from build123d import *

# Parameters (mm, degrees)
BOSS_EXTRUDE1_DEPTH     = 1.3
SKETCH2_R               = 1.33
CUT_EXTRUDE1_DEPTH      = 36.818151823
MIRROR2_COPY_1_SKETCH_R = 1.33
MIRROR2_COPY_1_DEPTH    = 36.818151823
CUT_EXTRUDE2_DEPTH      = 0.1
SKETCH4_R               = 0.5
CUT_EXTRUDE3_DEPTH      = 36.814661802
LPATTERN1_COUNT         = 20
LPATTERN1_PITCH         = 2.54
LPATTERN1_COUNT_DIR2    = 2
LPATTERN1_PITCH_DIR2    = 2.5
SKETCH5_R               = 0.5
CUT_EXTRUDE4_DEPTH      = 36.814661802
LPATTERN2_COUNT         = 2
LPATTERN2_PITCH         = 2.54
LPATTERN2_COUNT_DIR2    = 2
LPATTERN2_PITCH_DIR2    = 2.5
SKETCH7_R               = 3
CUT_EXTRUDE5_DEPTH      = 0.1
MIRROR4_COPY_1_SKETCH_R = 3
MIRROR4_COPY_1_DEPTH    = 0.1
SKETCH8_W               = 12
SKETCH8_H               = 12
BOSS_EXTRUDE2_DEPTH     = 1.25
BOSS_EXTRUDE3_START     = -7.8
BOSS_EXTRUDE3_DEPTH     = 7.6
CUT_EXTRUDE6_DEPTH      = 7.25
BOSS_EXTRUDE4_START     = -10.5
BOSS_EXTRUDE4_DEPTH     = 5.75
CUT_EXTRUDE7_DEPTH      = 5.4
LPATTERN3_COUNT         = 2
LPATTERN3_PITCH         = 12.5
BOSS_EXTRUDE5_START     = 29.3
SKETCH14_W              = 1.2
SKETCH14_H              = 17
BOSS_EXTRUDE5_DEPTH     = 4.1


with BuildPart() as part:
    # Sketch1 → Boss-Extrude1 (new body)
    with BuildSketch(Plane.XY):
        with BuildLine():
            Line((-29, -15), (29, -15))
            ThreePointArc((29, -15), (31.474873734, -13.974873734), (32.5, -11.5))
            Line((32.5, -11.5), (32.5, 11.5))
            ThreePointArc((32.5, 11.5), (31.474873734, 13.974873734), (29, 15))
            Line((29, 15), (-29, 15))
            ThreePointArc((-29, 15), (-31.474873734, 13.974873734), (-32.5, 11.5))
            Line((-32.5, 11.5), (-32.5, -11.5))
            ThreePointArc((-32.5, -11.5), (-31.474873734, -13.974873734), (-29, -15))
        make_face()
    extrude(amount=BOSS_EXTRUDE1_DEPTH)

    # Sketch2 → Cut-Extrude1 (cut, through all)
    with BuildSketch(Plane.XY.offset(1.3)):
        with Locations((-28.75, 11.25)):
            Circle(SKETCH2_R)
    cut_extrude1 = extrude(amount=-CUT_EXTRUDE1_DEPTH, mode=Mode.SUBTRACT)

    # Mirror1: Cut-Extrude1 across plane
    add(cut_extrude1.mirror(Plane.ZX), mode=Mode.SUBTRACT)

    # Mirror2: Cut-Extrude1 across plane
    add(cut_extrude1.mirror(Plane(origin=(0, 0, 0), x_dir=(0, 0, 1), z_dir=(1, 0, 0))), mode=Mode.SUBTRACT)

    # Mirror2 copy 1 sketch → Mirror2 copy 1 (cut, through all)
    with BuildSketch(Plane(origin=(0, 0, 1.3), x_dir=(-1, 0, 0), z_dir=(0, 0, 1))):
        with Locations((-28.75, 11.25)):
            Circle(MIRROR2_COPY_1_SKETCH_R)
    extrude(amount=-MIRROR2_COPY_1_DEPTH, mode=Mode.SUBTRACT)

    # Sketch3 → Cut-Extrude2 (cut)
    with BuildSketch(Plane.XY.offset(1.3)):
        Polygon((-25.5, 14.3), (25.5, 14.3), (25.5, 4.2), (20.4, 4.2), (20.4, 9.2), (-25.5, 9.2), align=None)
    extrude(amount=-CUT_EXTRUDE2_DEPTH, mode=Mode.SUBTRACT)

    # Sketch4 → Cut-Extrude3 (cut, through all)
    with BuildSketch(Plane.XY.offset(1.2)):
        with Locations((-24.13, 13)):
            Circle(SKETCH4_R)
    cut_extrude3 = extrude(amount=-CUT_EXTRUDE3_DEPTH, mode=Mode.SUBTRACT)

    # LPattern1: Cut-Extrude3 20 × 2
    with Locations(*[(i * LPATTERN1_PITCH, -j * LPATTERN1_PITCH_DIR2, 0) for i in range(LPATTERN1_COUNT) for j in range(LPATTERN1_COUNT_DIR2) if (i, j) != (0, 0)]):
        add(cut_extrude3, mode=Mode.SUBTRACT)

    # Sketch5 → Cut-Extrude4 (cut, through all)
    with BuildSketch(Plane.XY.offset(1.2)):
        with Locations((21.59, 8)):
            Circle(SKETCH5_R)
    cut_extrude4 = extrude(amount=-CUT_EXTRUDE4_DEPTH, mode=Mode.SUBTRACT)

    # LPattern2: Cut-Extrude4 2 × 2
    with Locations(*[(i * LPATTERN2_PITCH, -j * LPATTERN2_PITCH_DIR2, 0) for i in range(LPATTERN2_COUNT) for j in range(LPATTERN2_COUNT_DIR2) if (i, j) != (0, 0)]):
        add(cut_extrude4, mode=Mode.SUBTRACT)

    # Sketch7 → Cut-Extrude5 (cut)
    with BuildSketch(Plane.XY.offset(1.3)):
        with Locations((-28.75, 11.25)):
            Circle(SKETCH7_R)
    cut_extrude5 = extrude(amount=-CUT_EXTRUDE5_DEPTH, mode=Mode.SUBTRACT)

    # Mirror3: Cut-Extrude5 across plane
    add(cut_extrude5.mirror(Plane.ZX), mode=Mode.SUBTRACT)

    # Mirror4: Cut-Extrude5 across plane
    add(cut_extrude5.mirror(Plane(origin=(0, 0, 0), x_dir=(0, 0, 1), z_dir=(1, 0, 0))), mode=Mode.SUBTRACT)

    # Mirror4 copy 1 sketch → Mirror4 copy 1 (cut)
    with BuildSketch(Plane(origin=(0, 0, 1.3), x_dir=(-1, 0, 0), z_dir=(0, 0, 1))):
        with Locations((-28.75, 11.25)):
            Circle(MIRROR4_COPY_1_SKETCH_R)
    extrude(amount=-MIRROR4_COPY_1_DEPTH, mode=Mode.SUBTRACT)

    # Sketch8 → Boss-Extrude2 (add)
    with BuildSketch(Plane.XY.offset(1.3)):
        with Locations((-6.7, -2)):
            Rectangle(SKETCH8_W, SKETCH8_H)
    extrude(amount=BOSS_EXTRUDE2_DEPTH)

    # Sketch9 → Boss-Extrude3 (add)
    with BuildSketch(Plane(origin=(0, 0, 0), x_dir=(1, 0, 0), z_dir=(0, 1, 0)).offset(BOSS_EXTRUDE3_START)):
        Polygon((-24.175, -1.3), (-15.575, -1.3), (-14.25, -2.76), (-14.25, -4.6), (-25.5, -4.6), (-25.5, -2.76), align=None)
    extrude(amount=-BOSS_EXTRUDE3_DEPTH)

    # Sketch10 → Cut-Extrude6 (cut)
    with BuildSketch(Plane.XZ.offset(15.4)):
        Polygon((-14.6, 2.895140858), (-14.6, 4.25), (-25.15, 4.25), (-25.15, 2.895140858), (-24.01999203, 1.65), (-15.73000797, 1.65), align=None)
    extrude(amount=-CUT_EXTRUDE6_DEPTH, mode=Mode.SUBTRACT)

    # Sketch12 → Boss-Extrude4 (add)
    with BuildSketch(Plane(origin=(0, 0, 0), x_dir=(1, 0, 0), z_dir=(0, 1, 0)).offset(BOSS_EXTRUDE4_START)):
        Polygon((17.8, -3.9), (25.35, -3.9), (25.35, -2.57), (24.125, -1.3), (19.025, -1.3), (17.8, -2.57), align=None)
    boss_extrude4 = extrude(amount=-BOSS_EXTRUDE4_DEPTH)

    # Sketch13 → Cut-Extrude7 (cut)
    with BuildSketch(Plane.XZ.offset(16.25)):
        Polygon((18.15, 3.55), (18.15, 2.711290957), (19.173686159, 1.65), (23.976313841, 1.65), (25, 2.711290957), (25, 3.55), align=None)
    cut_extrude7 = extrude(amount=-CUT_EXTRUDE7_DEPTH, mode=Mode.SUBTRACT)

    # LPattern3: Boss-Extrude4, Cut-Extrude7 ×2
    with Locations(*[(-i * LPATTERN3_PITCH, 0, 0) for i in range(1, LPATTERN3_COUNT)]):
        add(boss_extrude4)
        add(cut_extrude7, mode=Mode.SUBTRACT)

    # Sketch14 → Boss-Extrude5 (add)
    with BuildSketch(Plane(origin=(0, 0, 0), x_dir=(0, 0, -1), z_dir=(1, 0, 0)).offset(BOSS_EXTRUDE5_START)):
        with Locations((-1.9, 0)):
            Rectangle(SKETCH14_W, SKETCH14_H)
    extrude(amount=BOSS_EXTRUDE5_DEPTH)


solid = part.part
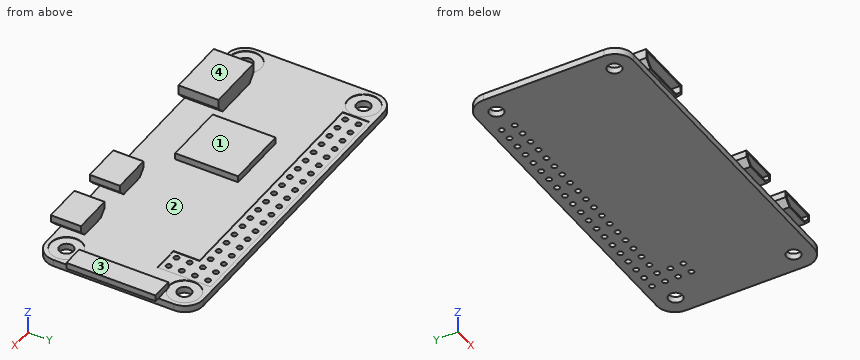
Model file for the job. Use its own axes, mm. Face numbers are marked on the shaded views. A direction names the side the tool comes from. Round coordinates to 2 decimals unless told otherwise and drop trailing zeros. Loops run counter-clockwise (first coordinate to the right, second up) from the corner with the lowest first, then second, coordinate; pieces in that order, holes last. Notation, with made-up numbers: M 72.5,42 L 89.5,42 A24 cw 89.5,65 Z; hole C 15,68.5 d11. An arc over 180 degrees is marked long. One line per question, with ' | ' between items.
1) Mould opens along X. For the marked faces 1 and 2 say: +X half, -X half, draft (parallel to the pull), parting line (faces both ways), or undercut.
Solved:
face 1: draft | face 2: undercut
2) Flat gauge pins, fed straight in: pin 1 (5 mm diameter, centred on x = 29.5, y = -12.5, fed in from +Z); pin 2 (1.3 mm diameter, centred on x = -17, z = 3, fed in from -Y); pin 3 (1.5 mm diameter, centred on y = -12, z = 3.5, fed in from -X). Where does each tip first touch, or does it go through?
Solved:
pin 1: stops at z = 1.3 | pin 2: stops at y = -8.15 | pin 3: stops at x = -25.5
3) Band-saw the part on A-A (y = 0.5). Give the cut face in (x, z).
Solved:
outline: M -32.5,0 L 32.5,0 L 32.5,1.3 L 33.4,1.3 L 33.4,2.5 L 29.3,2.5 L 29.3,1.3 L -0.7,1.3 L -0.7,2.55 L -12.7,2.55 L -12.7,1.3 L -32.5,1.3 Z
4) Drill centre lines: line 1 along Y through (x, z) = (8.89, 0.55); line 2 along Y through (x, z) = (28.75, 0.4); line 3 along Y through (x, z) = (24.13, 0.25). Where is each one in solid material? Low to high.
Solved:
line 1: y = -15 to 10, 11 to 12.5, 13.5 to 15 | line 2: y = -15 to -12.58, -9.92 to 9.92, 12.58 to 15 | line 3: y = -15 to 5, 6 to 7.5, 8.5 to 10, 11 to 12.5, 13.5 to 15
5) 3-axis set-ups, long thin cutter, end or side, ignore diameter. For the marked faces 3 and 4: which of +Z, -Z, +X, -X, +Y, -Y reach the whole face in a straight line?
Solved:
face 3: +Z, +X, +Y, -Y | face 4: +Z, +X, -X, +Y, -Y
